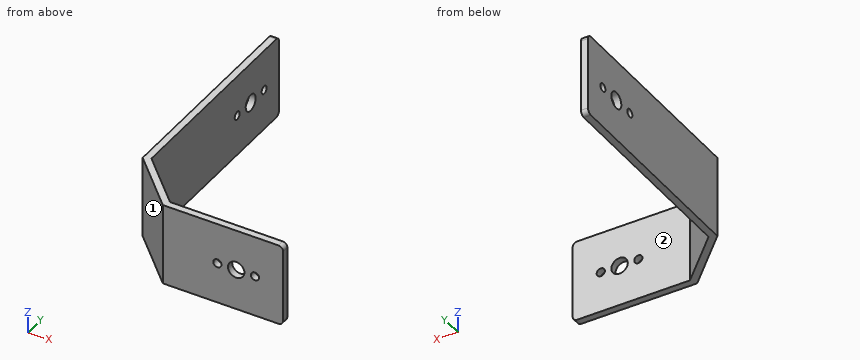
from build123d import *

# Parameters (mm, degrees)
EXTRU_MINCE1_DEPTH      = 35
ESQUISSE2_R             = 1.75
ESQUISSE2_R_2           = 3.5
ENL_V_MAT_EXTRU_1_DEPTH = 3
CONG_3_R                = 2
CONG_4_R                = 2
CONG_5_R                = 2
CONG_6_R                = 2
ESQUISSE3_R             = 1.75
ESQUISSE3_R_2           = 3.5
ENL_V_MAT_EXTRU_2_DEPTH = 10


with BuildPart() as part:
    # Esquisse1 → Extru.-Mince1 (new body)
    with BuildSketch(Plane.XY):
        Polygon((70, -20), (20, -20), (0, 0), (0, 90), (-3, 90), (-3, -1.242640687), (18.757359313, -23), (70, -23), align=None)
    extrude(amount=EXTRU_MINCE1_DEPTH)

    # Esquisse2 → Enlèv. mat.-Extru.1 (cut)
    with BuildSketch(Plane(origin=(0, 0, 0), x_dir=(0, 0, -1), z_dir=(1, 0, 0))):
        with Locations((-17.5, 79.5)):
            Circle(ESQUISSE2_R)
        with Locations((-17.5, 60.5)):
            Circle(ESQUISSE2_R)
        with Locations((-17.5, 70)):
            Circle(ESQUISSE2_R_2)
    extrude(amount=-ENL_V_MAT_EXTRU_1_DEPTH, mode=Mode.SUBTRACT)

    # Congé3
    cong_3_edges = [part.edges().sort_by_distance(p)[0] for p in [
        (-1.5, 90, 35),
    ]]
    fillet(cong_3_edges, radius=CONG_3_R)

    # Congé4
    cong_4_edges = [part.edges().sort_by_distance(p)[0] for p in [
        (-1.5, 90, 0),
    ]]
    fillet(cong_4_edges, radius=CONG_4_R)

    # Congé5
    cong_5_edges = [part.edges().sort_by_distance(p)[0] for p in [
        (70, -21.5, 35),
    ]]
    fillet(cong_5_edges, radius=CONG_5_R)

    # Congé6
    cong_6_edges = [part.edges().sort_by_distance(p)[0] for p in [
        (70, -21.5, 0),
    ]]
    fillet(cong_6_edges, radius=CONG_6_R)

    # Esquisse3 → Enlèv. mat.-Extru.2 (cut)
    with BuildSketch(Plane(origin=(0, -20, 0), x_dir=(1, 0, 0), z_dir=(0, 1, 0))):
        with Locations(Location((58, -17.5, 0), (0, 0, 270))):
            Circle(ESQUISSE3_R)
        with Locations(Location((42, -17.5, 0), (0, 0, 270))):
            Circle(ESQUISSE3_R)
        with Locations(Location((50, -17.5, 0), (0, 0, 270))):
            Circle(ESQUISSE3_R_2)
    extrude(amount=-ENL_V_MAT_EXTRU_2_DEPTH, mode=Mode.SUBTRACT)


solid = part.part
Geometry: final body of the model. Coordinates: model frame, mm. Face numbers are marked on the shaded views. A direction names the side the tool comes from. Round coordinates to 2 decimals unless told otherwise and drop trailing zeros. Loops run counter-clockwise (first coordinate to the right, second up) from the corner with the lowest first, then second, coordinate; pieces in that order, holes last. Notation, with made-up numbers: (3, 17) -> (20, 17) arc R22 ccw to (20, 51) -> close; hole circle Ø7 at (84.5, 48.25). An arc over 180 degrees is marked (long way). One line per question, with ' | ' between items. Start each with the question number.
1. Section D-D on z = 25. Output: boundary loops of the cut face in (x, y).
2. Set-up query: the marked faces 1 and 2. Return all of +Z, -Z, +X, -X, +Y, -Y with unobstructed straight access to the full face (end or side cutting, diameter ignored); none if empty.
3. Contact query for flat-ended pins moving along their axis: pin 1 (1 mm diameter, centred on x = 8.5, z = 26.5, fed in from -Y); pin 2 (3 mm diameter, centred on y = 33.5, z = 15, fed in from +X); pin 3 (12 mm diameter, centred on x = 52, z = 16, fed in from -Y); pin 4 (5.5 mm diameter, centred on x = 58, z = 17.5, fed in from +Y). Output: stop coordinate, or through.
4. Section B-B on x = 42. Output: boundary loops of the cut face in (y, z), and give its area (3 significant figures).
5. Line query: line 1 along Y through (x, z) = (-1.2, 17.5); line 2 along X through (y, z) = (4.5, 30.5); line 3 along Y through (x, z) = (64.5, 2.5). Output: solid intervals per line, ascending. Write a range as [from, to].
6. Section C-C on y = 60.5. Output: boundary loops of the cut face in (x, z), and give its area (3 significant figures).
7. Section A-A on z = 17.5. Count the separate pieces of the cut face and the enclosed holes in it, and give its area (3 significant figures).
Returned:
1) outline: (-3, -1.24) -> (18.76, -23) -> (70, -23) -> (70, -20) -> (20, -20) -> (0, 0) -> (0, 90) -> (-3, 90) -> close
2) face 1: +Z, -Z, -X, -Y | face 2: +Z, -Z, +X, +Y
3) pin 1: stops at y = -13.24 | pin 2: stops at x = 0 | pin 3: stops at y = -23 | pin 4: stops at y = -20
4) outline: (-23, 0) -> (-20, 0) -> (-20, 15.75) -> (-23, 15.75) -> close; (-23, 19.25) -> (-20, 19.25) -> (-20, 35) -> (-23, 35) -> close | area: 94.5 mm2
5) line 1: y = [-3.04, 58.75], [62.25, 66.5], [73.5, 77.75], [81.25, 90] | line 2: x = [-3, 0] | line 3: y = [-23, -20]
6) outline: (-3, 0) -> (0, 0) -> (0, 15.75) -> (-3, 15.75) -> close; (-3, 19.25) -> (0, 19.25) -> (0, 35) -> (-3, 35) -> close | area: 94.5 mm2
7) separate pieces: 7 | enclosed holes: 0 | area: 428 mm2
